CAD build for the part. Positions are in the model's coordinates, mm. Face numbers are marked on the shaded views. Round coordinates to 2 decimals unless told otherwise and drop trailing zeros. Loops run counter-clockwise (first coordinate to the right, second up) from the corner with the lowest first, then second, coordinate; pieces in that order, holes last. Notation, with made-up numbers: (58.25, 37.25) - (80.25, 37.25) arc R36 ccw to (80.25, 71.25) - close; hole circle Ø7 at (-31.5, -2.75). An arc over 180 degrees is marked (long way). Use one line per item in the form item = value.
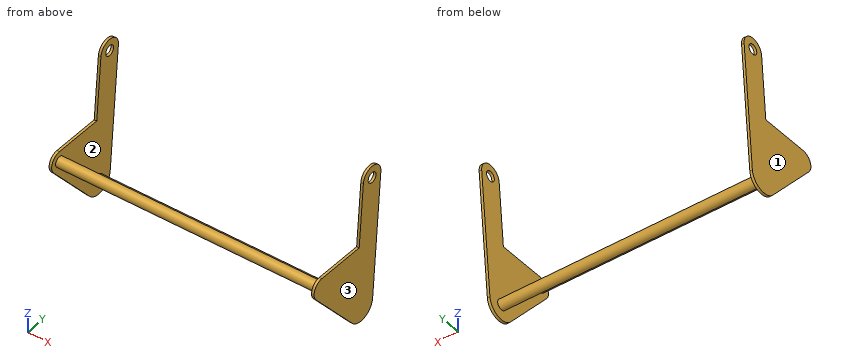
from build123d import *

# Parameters (mm, degrees)
BOSS_EXTRUDE1_DEPTH     = 660.4
SKETCH2_W               = 647.7
SKETCH2_H               = 371.475
CUT_EXTRUDE1_DEPTH      = 192.802928595
CUT_EXTRUDE1_DEPTH_BACK = 26.4
BOSS_EXTRUDE2_REACH     = 662.4
SKETCH3_R               = 12.7
SKETCH4_R               = 12.7
CUT_EXTRUDE2_DEPTH      = 1
CUT_EXTRUDE2_DEPTH_BACK = 661.4


with BuildPart() as part:
    # Sketch1 → Boss-Extrude1 (new body)
    with BuildSketch(Plane(origin=(0, 0, 0), x_dir=(0, 0, -1), z_dir=(1, 0, 0))):
        with BuildLine():
            Line((-180.290475349, 134.761665097), (-25.4, 121.210504416))
            Line((-25.4, 121.210504416), (-25.4, 0))
            ThreePointArc((-25.4, 0), (-10.544261728, -23.107975779), (16.645554694, -19.185554694))
            Line((16.645554694, -19.185554694), (151.968332041, 98.221667959))
            ThreePointArc((151.968332041, 98.221667959), (163.240880217, 138.756215424), (130.320633799, 164.955017997))
            Line((130.320633799, 164.955017997), (-175.309524651, 191.694192093))
            ThreePointArc((-175.309524651, 191.694192093), (-206.266263498, 165.718403944), (-180.290475349, 134.761665097))
        make_face()
    extrude(amount=BOSS_EXTRUDE1_DEPTH)

    # Sketch2 → Cut-Extrude1 (cut, two sides)
    with BuildSketch(Plane(origin=(0, 0, 0), x_dir=(1, 0, 0), z_dir=(0, 1, 0))) as cut_extrude1_sk:
        with Locations((330.2, -20.6375)):
            Rectangle(SKETCH2_W, SKETCH2_H)
    extrude(amount=CUT_EXTRUDE1_DEPTH, mode=Mode.SUBTRACT)
    extrude(cut_extrude1_sk.sketch, amount=-CUT_EXTRUDE1_DEPTH_BACK, mode=Mode.SUBTRACT)

    # Sketch3 → Boss-Extrude2 (add, up to next)
    with BuildSketch(Plane(origin=(660.4, 0, 0), x_dir=(0, 0, -1), z_dir=(1, 0, 0)), mode=Mode.PRIVATE) as boss_extrude2_sk1:
        with Locations((127, 127)):
            Circle(SKETCH3_R)
    boss_extrude2_tool1 = extrude(boss_extrude2_sk1.sketch, amount=-BOSS_EXTRUDE2_REACH, mode=Mode.PRIVATE) - part.part
    add(boss_extrude2_tool1.solids().sort_by_distance((660.4, 127, -127))[0])
    # Sketch3 → Boss-Extrude2 (add, up to next)
    with BuildSketch(Plane(origin=(660.4, 0, 0), x_dir=(0, 0, -1), z_dir=(1, 0, 0)), mode=Mode.PRIVATE) as boss_extrude2_sk2:
        Circle(SKETCH3_R)
    boss_extrude2_tool2 = extrude(boss_extrude2_sk2.sketch, amount=-BOSS_EXTRUDE2_REACH, mode=Mode.PRIVATE) - part.part
    add(boss_extrude2_tool2.solids().sort_by_distance((660.4, 0, 0))[0])

    # Sketch4 → Cut-Extrude2 (cut, two sides)
    with BuildSketch(Plane(origin=(660.4, 0, 0), x_dir=(0, 0, -1), z_dir=(1, 0, 0))) as cut_extrude2_sk:
        with Locations((-177.8, 163.227928595)):
            Circle(SKETCH4_R)
    extrude(amount=CUT_EXTRUDE2_DEPTH, mode=Mode.SUBTRACT)
    extrude(cut_extrude2_sk.sketch, amount=-CUT_EXTRUDE2_DEPTH_BACK, mode=Mode.SUBTRACT)


solid = part.part
1) Slice it at D-D (z = -123.5). Write the cut outline in (x, y).
Report:
outline = (0, 73.52) - (6.35, 73.52) - (6.35, 114.79) - (654.05, 114.79) - (654.05, 73.52) - (660.4, 73.52) - (660.4, 165.55) - (654.05, 165.55) - (654.05, 139.21) - (6.35, 139.21) - (6.35, 165.55) - (0, 165.55) - close
2) Slice it at B-B (z = 76.5). Write the cut outline in (x, y).
Report:
outline = (0, 125.68) - (6.35, 125.68) - (6.35, 183.05) - (0, 183.05) - close; (654.05, 125.68) - (660.4, 125.68) - (660.4, 183.05) - (654.05, 183.05) - close
3) Slice it at C-C (y = 20.5). Write the cut outline in (x, z), plus the area to 3 significant figures.
Report:
outline = (0, -62.39) - (6.35, -62.39) - (6.35, 25.4) - (0, 25.4) - close; (654.05, -62.39) - (660.4, -62.39) - (660.4, 25.4) - (654.05, 25.4) - close
area = 1,110 mm^2
4) Slice it at A-A (x = 476). Write the cut outline in (y, z).
Report:
outline = circle Ø25.4 at (0, 0); circle Ø25.4 at (127, -127)
5) Drill centre lines: probe 1 along X at (y, z) = (127, 83.5); probe 2 along Y at (x, z) = (2.75, 177.8). Where is each one in solid material? Low to high.
Report:
probe_1 = 0 to 6.35, 654.05 to 660.4
probe_2 = 134.54 to 150.53, 175.93 to 191.8
6) Flat gauge pins, fed straight in: pin 1 (5 mm diameter, centred on x = 106, y = 128.5, fed in from -Z); pin 2 (10 mm diameter, centred on x = 371.5, y = 15.5, fed in from -Z); pin 3 (1.9 mm diameter, centred on x = 3, y = 36, fed in from +Z). Where does each tip first touch, or does it go through?
Report:
pin_1 = -139.7
pin_2 = -7.14
pin_3 = 25.4
7) Two-plate mould, pull along X, no slides. Class the marked faces 1, 2 and 3: +X half, -X half, draft (parallel to the pull), parting line (faces both ways), or undercut.
Report:
face_1 = -X half
face_2 = undercut
face_3 = +X half
